```python
from build123d import *

# Parameters (mm, degrees)
SKETCH1_R           = 8.763
BOSS_EXTRUDE1_DEPTH = 3.556
BOSS_EXTRUDE2_DEPTH = 19.05
SKETCH3_R           = 9.906
CUT_EXTRUDE1_DEPTH  = 17.78
SKETCH4_R           = 6.35
CUT_EXTRUDE2_DEPTH  = 17.78
SKETCH5_W           = 10.287
SKETCH5_H           = 10.16
CUT_EXTRUDE3_DEPTH  = 12.7


with BuildPart() as part:
    # Sketch1 → Boss-Extrude1 (new body)
    with BuildSketch(Plane.XY):
        with BuildLine():
            Line((11.938, 0), (11.938, -11.938))
            Line((11.938, -11.938), (22.225, -11.938))
            Line((22.225, -11.938), (22.225, -17.78))
            Line((22.225, -17.78), (-22.225, -17.78))
            Line((-22.225, -17.78), (-22.225, -11.938))
            Line((-22.225, -11.938), (-11.938, -11.938))
            Line((-11.938, -11.938), (-11.938, 0))
            ThreePointArc((-11.938, 0), (0, 11.938), (11.938, 0))
        make_face()
        Circle(SKETCH1_R, mode=Mode.SUBTRACT)
    extrude(amount=BOSS_EXTRUDE1_DEPTH)

    # Sketch2 → Boss-Extrude2 (add)
    with BuildSketch(Plane.XY.offset(3.556)):
        with BuildLine():
            Line((-11.938, 0), (-11.938, -11.938))
            Line((-11.938, -11.938), (-22.225, -11.938))
            Line((-22.225, -11.938), (-22.225, -17.78))
            Line((-22.225, -17.78), (22.225, -17.78))
            Line((22.225, -17.78), (22.225, -11.938))
            Line((22.225, -11.938), (11.938, -11.938))
            Line((11.938, -11.938), (11.938, 0))
            ThreePointArc((11.938, 0), (0, 11.938), (-11.938, 0))
        make_face()
    extrude(amount=BOSS_EXTRUDE2_DEPTH)

    # Sketch3 → Cut-Extrude1 (cut)
    with BuildSketch(Plane.XY.offset(22.606)):
        Circle(SKETCH3_R)
    extrude(amount=-CUT_EXTRUDE1_DEPTH, mode=Mode.SUBTRACT)

    # Sketch4 → Cut-Extrude2 (cut)
    with BuildSketch(Plane.XY.offset(4.826)):
        Circle(SKETCH4_R)
    extrude(amount=-CUT_EXTRUDE2_DEPTH, mode=Mode.SUBTRACT)

    # Sketch5 → Cut-Extrude3 (cut)
    with BuildSketch(Plane(origin=(0, -11.938, 0), x_dir=(1, 0, 0), z_dir=(0, 1, 0))):
        with Locations((17.0815, -5.08)):
            Rectangle(SKETCH5_W, SKETCH5_H)
        with Locations((-17.0815, -5.08)):
            Rectangle(SKETCH5_W, SKETCH5_H)
    extrude(amount=-CUT_EXTRUDE3_DEPTH, mode=Mode.SUBTRACT)


solid = part.part
```
Verification items for the finished model (mm, model axes). A direction names the side the tool comes from. Give positions to 0.01 mm unless a question says otherwise; leave off trailing zeros. Write each loop counter-clockwise with the first axis right and the second up, starting at its lowest first coordinate (ties: lowest second). Pieces come first, ordered by that corner, then holes. Notation, with made-up numbers: (60, 82) - (95, 82) arc R26 cw to (95, 112) - close; hole circle Ø4 at (0, 71.25). An arc over 180 degrees is marked (long way). Put each result on its own line as item: value.
Q1. Set-up check for faces 1 (the face through (-17, -15, 10.16)), 2 (the face through (6, 3, 3.556)), 3 (the face through (-0.1, -6.5, 4.826)): record each of +Z, -Z, +X, -X, +Y, -Y from which the full face is reachable in a straight line by a thin tool's end or side.
Result:
face 1: -Z, -X, +Y, -Y
face 2: -Z
face 3: +Z
Q2. Section check C-C on y = -1.75. Record the cut outline in (x, z).
Result:
outline: (-11.94, 0) - (-8.59, 0) - (-8.59, 3.56) - (-6.1, 3.56) - (-6.1, 4.83) - (-9.75, 4.83) - (-9.75, 22.61) - (-11.94, 22.61) - close; (6.1, 3.56) - (8.59, 3.56) - (8.59, 0) - (11.94, 0) - (11.94, 22.61) - (9.75, 22.61) - (9.75, 4.83) - (6.1, 4.83) - close
Q3. Mould release check, pull along X, two halves, no side actions. Record for faces 4 (the face through (0.263, 11.935, 11.145)), 5 (the face through (-1.38, -6.2, 4.2)), 6 (the face through (-22.225, -15, 16)), 7 (the face through (8.36, 2.63, 1.75)): released by +X, released by -X, zero draft, split by the parting line, or undercut.
Result:
face 4: split by the parting line
face 5: undercut
face 6: released by -X
face 7: undercut
Q4. Section check A-A on x = 0. Record the cut outline in (y, z).
Result:
outline: (-17.78, 0) - (-8.76, 0) - (-8.76, 3.56) - (-6.35, 3.56) - (-6.35, 4.83) - (-9.91, 4.83) - (-9.91, 22.61) - (-17.78, 22.61) - close; (6.35, 3.56) - (8.76, 3.56) - (8.76, 0) - (11.94, 0) - (11.94, 22.61) - (9.91, 22.61) - (9.91, 4.83) - (6.35, 4.83) - close
Q5. Section check B-B on z = 11.25. Record the cut outline in (x, y) (3 decimals), and give its area (3 significant figures).
Result:
outline: (-22.225, -17.78) - (22.225, -17.78) - (22.225, -11.938) - (11.938, -11.938) - (11.938, 0) arc R11.938 ccw to (-11.938, 0) - (-11.938, -11.938) - (-22.225, -11.938) - close; hole circle Ø19.812 at (0, 0)
area: 460 mm2
Q6. Scan lines: probe 1 along Y at (x, z) = (0, 2.7); probe 2 along Y at (x, z) = (0, 17.5); probe 3 along X at (y, z) = (-2, 20.75). Record each from-to range of solid material in increasing order. Write a range as from..to.
Result:
probe 1: -17.78..-8.76, 8.76..11.94
probe 2: -17.78..-9.91, 9.91..11.94
probe 3: -11.94..-9.7, 9.7..11.94
Q7. Section check D-D on y = -7.75. Record the cut outline in (x, z), and give its area (3 significant figures).
Result:
outline: (-11.94, 0) - (-4.09, 0) - (-4.09, 3.56) - (4.09, 3.56) - (4.09, 0) - (11.94, 0) - (11.94, 22.61) - (6.17, 22.61) - (6.17, 4.83) - (-6.17, 4.83) - (-6.17, 22.61) - (-11.94, 22.61) - close
area: 291 mm2
Q8. Depth check by flat-ended pin: P1, Ø8, axis at x = -16.5, z = 19.5, coming from the +Y side; P2, Ø8, axis at y = 0, z = 19.5, coming from the -X side; P3, Ø4, axis at y = 1.5, z = 11.5, coming from the +X side; P4, Ø7.5, axis at x = 0, y = 0, coming from the +Z side. Enter the tip coordinate at first touch or a pass-through.
Result:
P1: y = -11.94
P2: x = -11.94
P3: x = 11.94
P4: through
